Here's how the part is built. I have some questions about the finished solid (model axes, mm). Face numbers are marked on the shaded views. Coordinates: 2 decimals unless noted, no trailing zeros. Write each loop counter-clockwise with the first axis right and the second up, starting at its lowest first coordinate (ties: lowest second). Pieces come first, ordered by that corner, then holes. Notation, with made-up numbers: M -11,-8.5 L 4,-8.5 A13 cw 4,12.5 Z; hole C 49,-10 d5. An arc over 180 degrees is marked long. Use a Markdown table: item, result.
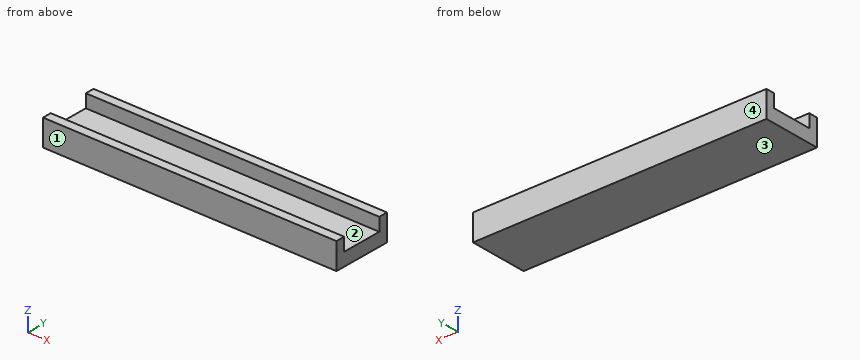
```python
from build123d import *

# Parameters (mm, degrees)
F0_W     = 90
F0_H     = 2.75
F1_DEPTH = 8
F0_H_2   = 12.5
F2_DEPTH = 4


with BuildPart() as f1:
    # F0 (on Top) → F1 (new body)
    with BuildSketch(Plane.XY):
        with Locations((0, 7.625)):
            Rectangle(F0_W, F0_H)
    extrude(amount=F1_DEPTH)



with BuildPart() as f1b:
    # F0 (on Top) → F1, piece 2 (new body)
    with BuildSketch(Plane.XY):
        with Locations((0, -7.625)):
            Rectangle(F0_W, F0_H)
    extrude(amount=F1_DEPTH)


with BuildPart() as f1_1:
    add(f1.part)

    add(f1b.part)  # F2 merges F1b
    # F0 (on Top) → F2 (join)
    with BuildSketch(Plane.XY):
        Rectangle(F0_W, F0_H_2)
    extrude(amount=F2_DEPTH)


solid = f1_1.part
```
1. We'd pull the mould along Y, two halves only. Please class the marked faces 1, 2, 3 and 4: +Y half, -Y half, draft (parallel to the pull), parting line (faces both ways), or undercut.
Answers follow:
| item | result |
|---|---|
| face 1 | -Y half |
| face 2 | undercut |
| face 3 | draft |
| face 4 | +Y half |
2. Suppose I cut it at C-C on y = -3.5. Write out the boundary of the cut face in (x, z), and give its area (3 significant figures).
Answers follow:
| item | result |
|---|---|
| outline | M -45,0 L 45,0 L 45,4 L -45,4 Z |
| area | 360 mm2 |
3. Will this pin go through, and if not, where does the flat tip stop? pin 1 Ø5 at (x, y) = (-29, -2) entering from +Z.
Answers follow:
| item | result |
|---|---|
| pin 1 | stops at z = 4 |
4. Suppose I cut it at B-B on x = 35. Write out the boundary of the cut face in (y, z).
Answers follow:
| item | result |
|---|---|
| outline | M -9,0 L 9,0 L 9,8 L 6.25,8 L 6.25,4 L -6.25,4 L -6.25,8 L -9,8 Z |
5. I need wall thicknesses on probe 1 along Y at (x, z) = (-29.5, 5.75); probe 2 along Z at (x, y) = (3, 1). Which ranges of each line are inside material? Lowest first, please.
Answers follow:
| item | result |
|---|---|
| probe 1 | y = -9 to -6.25, 6.25 to 9 |
| probe 2 | z = 0 to 4 |
6. Suppose I cut it at A-A on z = 5. Write out the boundary of the cut face in (x, y).
Answers follow:
| item | result |
|---|---|
| outline | M -45,-9 L 45,-9 L 45,-6.25 L -45,-6.25 Z; M -45,6.25 L 45,6.25 L 45,9 L -45,9 Z |
